```python
from build123d import *

# Parameters (mm, degrees)
SKETCH1_W           = 80
SKETCH1_H           = 80
BOSS_EXTRUDE1_DEPTH = 32
SKETCH3_R           = 5.375
CUT_EXTRUDE1_DEPTH  = 95.994736856
CHAMFER1_SIZE       = 15
SKETCH4_R           = 3.5
CUT_EXTRUDE2_DEPTH  = 7.5
SKETCH5_R           = 9
CUT_EXTRUDE3_DEPTH  = 93.482430925


with BuildPart() as part:
    # Sketch1 → Boss-Extrude1 (new body)
    with BuildSketch(Plane(origin=(0, 0, 0), x_dir=(1, 0, 0), z_dir=(0, 1, 0))):
        Rectangle(SKETCH1_W, SKETCH1_H)
    extrude(amount=BOSS_EXTRUDE1_DEPTH)

    # Sketch2 → Cut-Revolve1 (revolve, cut)
    with BuildSketch(Plane(origin=(0, 32, 0), x_dir=(1, 0, 0), z_dir=(0, 1, 0))):
        with BuildLine():
            Line((-33, 0), (33, 0))
            ThreePointArc((33, 0), (0, -30), (-33, 0))
        make_face()
    revolve(axis=Axis((-33, 32, 0), (1, 0, 0)), mode=Mode.SUBTRACT)

    # Sketch3 → Cut-Extrude1 (cut, through all)
    with BuildSketch(Plane.ZY.offset(40)):
        with Locations((0, 32)):
            Circle(SKETCH3_R)
    extrude(amount=-CUT_EXTRUDE1_DEPTH, mode=Mode.SUBTRACT)

    # Chamfer1
    chamfer1_edges = [part.edges().sort_by_distance(p)[0] for p in [
        (40, 16, 40),
        (-40, 16, 40),
        (-40, 16, -40),
        (40, 16, -40),
    ]]
    chamfer(chamfer1_edges, length=CHAMFER1_SIZE)

    # Sketch4 → Cut-Extrude2 (cut)
    with BuildSketch(Plane(origin=(0, 32, 0), x_dir=(1, 0, 0), z_dir=(0, 1, 0))):
        with Locations(Location((-27.5, 27.5, 0), (0, 0, 270))):
            Circle(SKETCH4_R)
        with Locations(Location((27.5, 27.5, 0), (0, 0, 270))):
            Circle(SKETCH4_R)
        with Locations(Location((27.5, -27.5, 0), (0, 0, 270))):
            Circle(SKETCH4_R)
        with Locations(Location((-27.5, -27.5, 0), (0, 0, 270))):
            Circle(SKETCH4_R)
    extrude(amount=-CUT_EXTRUDE2_DEPTH, mode=Mode.SUBTRACT)

    # Sketch5 → Cut-Extrude3 (cut, through all)
    with BuildSketch(Plane.ZY.offset(37)):
        with Locations((0, 32)):
            Circle(SKETCH5_R)
    cut_extrude3 = extrude(amount=CUT_EXTRUDE3_DEPTH, mode=Mode.SUBTRACT)

    # Mirror1: Cut-Extrude3 across plane
    add(cut_extrude3.mirror(Plane(origin=(0, 0, 0), x_dir=(0, 0, 1), z_dir=(1, 0, 0))), mode=Mode.SUBTRACT)


solid = part.part
```
Input: part model. Units: mm. Frame: model coordinates. A direction names the side the tool comes from. Coordinates: 2 decimals unless noted, no trailing zeros.
1) Pin query (flat end, axial travel): pin 1 Ø6 at (x, z) = (14, -27) entering from -Y; pin 2 Ø2 at (x, z) = (27.5, -26) entering from +Y; pin 3 Ø1 at (x, y) = (-31, 25.5) entering from -Z. Return the tip coordinate at first contact, or that it passes through.
2) Material intervals for line 1 along Z through (x, y) = (27, 26); line 2 along X through (y, z) = (28, -27); line 3 along X through (y, z) = (15, 13.5), sorted ascending.
3) Section A-A on y = 30. State how many separate pieces and enclosed holes the cut face has, and give its area (3 significant figures).
4) Mould query, pull axis Z, two halves, no side actions, for faces 4 (the cylindrical face through (30.45, 28.3, -25.62)), 5 (the flat face through (40, 16, 0)), 6 (the cylindrical face through (38, 23, 0)), 7 (the flat face through (-32, 16, -33)). Classes: pulls with the +Z half, pulls with the -Z half, needs draft (parallel to the pull), parting line crosses it, or undercut.
5) Set-up query: faces 1 (the cylindrical face through (-38, 23, 0)), 2 (the flat face through (37, 26, 0)), 3 (the flat face through (-27, 24.5, -28)). Return all of +Z, -Z, +X, -X, +Y, -Y with unobstructed straight access to the full face (end or side cutting, diameter ignored); none if empty.
Check result:
1. pin 1: stops at y = 0
1. pin 2: stops at y = 24.5
1. pin 3: stops at z = -34.5
2. line 1: z = -38 to -30.96, -24.04 to -14.92, 14.92 to 24.04, 30.96 to 38
2. line 2: x = -38 to -30.96, -24.04 to -13.12, 13.12 to 24.04, 30.96 to 38
2. line 3: x = -40 to -21.93, 21.93 to 40
3. separate pieces: 2
3. enclosed holes: 4
3. area: 2,580 mm2
4. face 4: undercut
4. face 5: needs draft
4. face 6: undercut
4. face 7: pulls with the -Z half
5. face 1: -X, +Y
5. face 2: +X, +Y
5. face 3: +Y
